For this review, take the finished solid that the model builds, in its own axes (mm). A direction names the side the tool comes from. Round coordinates to 2 decimals unless told otherwise and drop trailing zeros. Loops run counter-clockwise (first coordinate to the right, second up) from the corner with the lowest first, then second, coordinate; pieces in that order, holes last. Notation, with made-up numbers: M -6.5,39 L 20.5,39 A8 ccw 20.5,46 Z; hole C 47.25,37.25 d8. An arc over 180 degrees is marked long. One line per question, with ' | ' between items. Start each with the question number.
1) For pin 1 Ø3 at (x, y) = (31, 15) entering from +Z, flat-tipped, find the tip position at first contact; note if it passes through.
2) For probe 1 along Y at (x, z) = (-31.5, 76.5); probe 2 along X at (y, z) = (-12, -159); probe 3 along Y at (x, z) = (39.2, 0), list the stretches that pass through material, from the lowest coordinate up. Write a range as from..to.
3) We need section A-A (x = 8.5). Give the boundary of the cut face in (y, z), and give its area (3 significant figures).
4) Mouldability with a two-part tool opening along Y and no side actions: class faces 1 (the face through (-3, -18, -208)), 2 (the face through (0, 20, 3)), 3 (the face through (38.479, 7.214, -0.553)) as pulls with the +Y half, pulls with the -Y half, needs draft (parallel to the pull), parting line crosses it, or undercut.
5) We need section D-D (z = 0). Give the boundary of the cut face in (x, y).
6) We need section B-B (y = 3). Give the boundary of the cut face in (x, z), and give its area (3 significant figures).
7) For faces 4 (the face through (37, -4, 3)), 5 (the face through (0, -20, 3)), list the 3-axis set-ups (+Z, -Z, +X, -X, +Y, -Y) from which the entire face can be reached by the end or side of a thin tool; tool diameter is ignored.
8) We need section C-C (z = 80.5). Give the boundary of the cut face in (x, y).
```python
from build123d import *

# Parameters (mm, degrees)
EXTRUDE_1_DEPTH        = 208
HOLE_WIZARD_M101_D     = 8.5
HOLE_WIZARD_M101_DEPTH = 27.5
HOLE_WIZARD_M101_TIP   = 2.553657631


with BuildPart() as part:
    # Эскиз1 → Бобышка-Вытянуть1 (new, symmetric)
    with BuildSketch(Plane.XY):
        with BuildLine():
            Line((-35, -20), (35, -20))
            ThreePointArc((35, -20), (38.535533906, -18.535533906), (40, -15))
            Line((40, -15), (40, 15))
            ThreePointArc((40, 15), (38.535533906, 18.535533906), (35, 20))
            Line((35, 20), (-35, 20))
            ThreePointArc((-35, 20), (-38.535533906, 18.535533906), (-40, 15))
            Line((-40, 15), (-40, -15))
            ThreePointArc((-40, -15), (-38.535533906, -18.535533906), (-35, -20))
        make_face()
        with BuildLine():
            Line((-35, -17), (35, -17))
            ThreePointArc((35, -17), (36.414213562, -16.414213562), (37, -15))
            Line((37, -15), (37, 15))
            ThreePointArc((37, 15), (36.414213562, 16.414213562), (35, 17))
            Line((35, 17), (-35, 17))
            ThreePointArc((-35, 17), (-36.414213562, 16.414213562), (-37, 15))
            Line((-37, 15), (-37, -15))
            ThreePointArc((-37, -15), (-36.414213562, -16.414213562), (-35, -17))
        make_face(mode=Mode.SUBTRACT)
    extrude(amount=EXTRUDE_1_DEPTH, both=True)

    # Отверстие обработанное метчиком M101
    with Locations(Plane(origin=(40, 0, 0), x_dir=(0, 0, -1), z_dir=(1, 0, 0))):
        with Locations((400, 3), (0, 3), (-400, 3)):
            Hole(HOLE_WIZARD_M101_D / 2, depth=HOLE_WIZARD_M101_DEPTH)
            with Locations((0, 0, -(HOLE_WIZARD_M101_DEPTH + HOLE_WIZARD_M101_TIP / 2))):  # 118° drill point
                Cone(0, HOLE_WIZARD_M101_D / 2, HOLE_WIZARD_M101_TIP, mode=Mode.SUBTRACT)


solid = part.part
```
Answers below:
1) pin 1: through
2) probe 1: -20..-17, 17..20 | probe 2: -40..-37, 37..40 | probe 3: -17.71..-1.25, 7.25..17.71
3) outline: M -20,-208 L -17,-208 L -17,208 L -20,208 Z; M 17,-208 L 20,-208 L 20,208 L 17,208 Z | area: 2,500 mm^2
4) face 1: needs draft | face 2: pulls with the +Y half | face 3: undercut
5) outline: M -40,-15 A5 ccw -35,-20 L 35,-20 A5 ccw 40,-15 L 40,-1.25 L 37,-1.25 L 37,-15 A2 cw 35,-17 L -35,-17 A2 cw -37,-15 L -37,15 A2 cw -35,17 L 35,17 A2 cw 37,15 L 37,7.25 L 40,7.25 L 40,15 A5 ccw 35,20 L -35,20 A5 ccw -40,15 Z
6) outline: M -40,-208 L -37,-208 L -37,208 L -40,208 Z; M 37,-208 L 40,-208 L 40,-4.25 L 37,-4.25 Z; M 37,4.25 L 40,4.25 L 40,208 L 37,208 Z | area: 2,470 mm^2
7) face 4: +Z, -Z | face 5: +Z, -Z, +X, -X, -Y
8) outline: M -40,-15 A5 ccw -35,-20 L 35,-20 A5 ccw 40,-15 L 40,15 A5 ccw 35,20 L -35,20 A5 ccw -40,15 Z; hole M -37,-15 A2 ccw -35,-17 L 35,-17 A2 ccw 37,-15 L 37,15 A2 ccw 35,17 L -35,17 A2 ccw -37,15 Z
